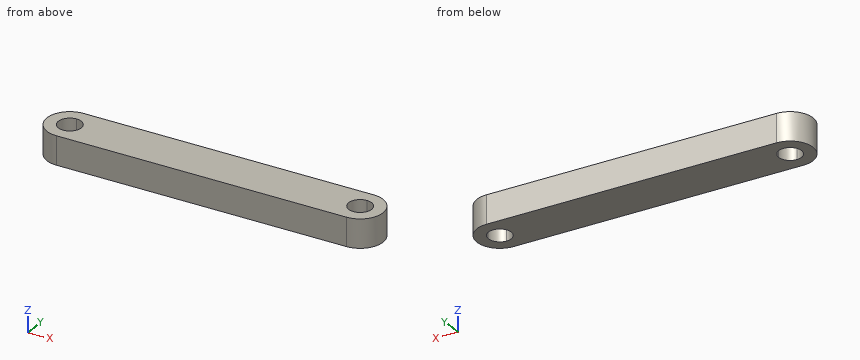
```python
from build123d import *

# Parameters (mm, degrees)
F1_DEPTH = 3.175


with BuildPart() as f1:
    # F0 (on Top) → F1 (new body)
    with BuildSketch(Plane.XY):
        with BuildLine():
            Line((15.875, 1.27), (15.875, 2.54))
            Line((15.875, 2.54), (-15.875, 2.54))
            Line((-15.875, 2.54), (-15.875, 1.27))
            ThreePointArc((-15.875, 1.27), (-14.976974, 0.898026), (-14.605, 0))
            ThreePointArc((-14.605, 0), (-14.976974, -0.898026), (-15.875, -1.27))
            Line((-15.875, -1.27), (-15.875, -2.54))
            Line((-15.875, -2.54), (15.875, -2.54))
            Line((15.875, -2.54), (15.875, -1.27))
            ThreePointArc((15.875, -1.27), (14.605, 0), (15.875, 1.27))
        make_face()
        with BuildLine():
            ThreePointArc((15.875, -2.54), (18.415, 0), (15.875, 2.54))
            Line((15.875, 2.54), (15.875, 1.27))
            ThreePointArc((15.875, 1.27), (16.773026, 0.898026), (17.145, 0))
            ThreePointArc((17.145, 0), (16.773026, -0.898026), (15.875, -1.27))
            Line((15.875, -1.27), (15.875, -2.54))
        make_face()
        with BuildLine():
            Line((-15.875, 1.27), (-15.875, 2.54))
            ThreePointArc((-15.875, 2.54), (-18.415, 0), (-15.875, -2.54))
            Line((-15.875, -2.54), (-15.875, -1.27))
            ThreePointArc((-15.875, -1.27), (-17.145, 0), (-15.875, 1.27))
        make_face()
    extrude(amount=F1_DEPTH)


solid = f1.part
```
Can you work these out from the model? Positions are in its coordinate system, mm. Give positions to 0.01 mm unless a question says otherwise; leave off trailing zeros. Write each loop counter-clockwise with the first axis right and the second up, starting at its lowest first coordinate (ties: lowest second). Pieces come first, ordered by that corner, then holes. Notation, with made-up numbers: (48.25, 14.25) -> (72.25, 14.25) arc R20 ccw to (72.25, 27.25) -> close; hole circle Ø8 at (31.25, 29). An arc over 180 degrees is marked (long way). Write item = value, one per line.
(1) Suppose I cut it at B-B on z = 1.1. Write out the boundary of the cut face in (x, y) (3 decimals).
Worked out:
outline = (-15.875, -2.54) -> (15.875, -2.54) arc R2.54 ccw to (15.875, 2.54) -> (-15.875, 2.54) arc R2.54 ccw to start; hole (-15.875, -1.27) arc R1.27 ccw to (-14.605, 0) arc R1.27 ccw to (-15.875, 1.27) arc R1.27 ccw to start; hole (15.875, -1.27) arc R1.27 ccw to (17.145, 0) arc R1.27 ccw to (15.875, 1.27) arc R1.27 ccw to start
(2) I need wall thicknesses on probe 1 along Y at (x, z) = (16, 0.75); probe 2 along X at (y, z) = (0.45, 1.9); probe 3 along X at (y, z) = (-0.55, 1.7). Which ranges of each line are inside material? Lowest first, please. Write a range as from..to.
Worked out:
probe_1 = -2.54..-1.26, 1.26..2.54
probe_2 = -18.37..-17.06, -14.69..14.69, 17.06..18.37
probe_3 = -18.35..-17.02, -14.73..14.73, 17.02..18.35
(3) I'm going to push flat-ended pins straight in: P1, Ø1.5, axis at x = 5, y = 1, coming from the -Z side; P2, Ø1.5, axis at y = -1, z = 0.5, coming from the -X side. Where does each tip first touch, or does it pass through?
Worked out:
P1 = 0
P2 = -18.4
(4) Suppose I cut it at A-A on y = 0.7. Write out the boundary of the cut face in (x, z) (3 decimals), then the cut area to 3 significant figures.
Worked out:
outline = (-18.317, 0) -> (-16.935, 0) -> (-16.935, 3.175) -> (-18.317, 3.175) -> close; (-14.815, 0) -> (14.815, 0) -> (14.815, 3.175) -> (-14.815, 3.175) -> close; (16.935, 0) -> (18.317, 0) -> (18.317, 3.175) -> (16.935, 3.175) -> close
area = 103 mm^2
